Check sheet for the modelled part. Datum: model origin and axes. Units: mm. A direction names the side the tool comes from. Give positions to 0.01 mm unless a question says otherwise; leave off trailing zeros. Write each loop counter-clockwise with the first axis right and the second up, starting at its lowest first coordinate (ties: lowest second). Pieces come first, ordered by that corner, then holes. Notation, with made-up numbers: (26, 5) -> (81, 5) arc R17 cw to (81, 29) -> close; hole circle Ø6 at (88, 51). An arc over 180 degrees is marked (long way). Answer as a JSON object with one key per item and string values.
from build123d import *

# Parameters (mm, degrees)
F0_W     = 162.56
F0_H     = 120.65
F1_DEPTH = 6.35
F2_W     = 162.56
F2_H     = 120.65
F2_W_2   = 149.86
F2_H_2   = 107.95
F3_DEPTH = 6.35
F4_R     = 5.08


with BuildPart() as f1:
    # F0 (on Top) → F1 (new body)
    with BuildSketch(Plane.XY):
        with Locations((17.590381, -7.976995)):
            Rectangle(F0_W, F0_H)
    extrude(amount=F1_DEPTH)

    # F2 (on face) → F3 (join)
    with BuildSketch(Plane.XY.offset(6.35)):
        with Locations((17.590381, -7.976995)):
            Rectangle(F2_W, F2_H)
        with Locations((17.590381, -7.976995)):
            Rectangle(F2_W_2, F2_H_2, mode=Mode.SUBTRACT)
    extrude(amount=F3_DEPTH)

    # F4
    f4_edges = [f1.edges().sort_by_distance(p)[0] for p in [
        (98.870381, -68.301995, 6.35),
        (98.870381, 52.348005, 6.35),
        (-63.689619, 52.348005, 6.35),
        (-63.689619, -68.301995, 6.35),
    ]]
    fillet(f4_edges, radius=F4_R)


solid = f1.part
1. Scan lines: L1, parallel to X at y = -48.5, z = 7.5; L2, parallel to Y at x = 11.5, z = 12; L3, parallel to Z at x = 60, y = -47. Record each from-to range of solid material in increasing order. Write a range as [from, to].
Determined:
{"L1": "[-63.69, -57.34], [92.52, 98.87]", "L2": "[-68.3, -61.95], [46, 52.35]", "L3": "[0, 6.35]"}
2. Mould release check, pull along X, two halves, no side actions. Record for faces 1 (the face through (11, -66, 12.7)), 2 (the face through (-62.241, -66.774, 6.439)), 3 (the face through (92.52, -9, 9)): released by +X, released by -X, zero draft, split by the parting line, or undercut.
Determined:
{"face 1": "zero draft", "face 2": "released by -X", "face 3": "undercut"}
3. Go/stop test with a flat-tipped pin: P1, Ø2, axis at x = -25, y = 35, coming from the +Z side. Record where the tip stops, or that it passes through.
Determined:
{"P1": "z = 6.35"}
4. Access from +Z, -Z, +X, -X, +Y, -Y to the whole of each face (thin tool, end or side, straight path). Record for faces 4 (the face through (17, -61.952, 9)), 5 (the face through (17, 52.348, 6)).
Determined:
{"face 4": "+Z", "face 5": "+Z, -Z, +X, -X, +Y"}
5. Sectioned sample at C-C, the plane y = 24.5. Enter the section's corners in (x, z).
Determined:
{"outline": "(-63.69, 0) -> (98.87, 0) -> (98.87, 12.7) -> (92.52, 12.7) -> (92.52, 6.35) -> (-57.34, 6.35) -> (-57.34, 12.7) -> (-63.69, 12.7) -> close"}
6. Sectioned sample at A-A, the plane z = 8.25. Enter the section's corners in (x, y), plus the area to 3 significant figures.
Determined:
{"outline": "(-63.69, -63.22) arc R5.08 ccw to (-58.61, -68.3) -> (93.79, -68.3) arc R5.08 ccw to (98.87, -63.22) -> (98.87, 47.27) arc R5.08 ccw to (93.79, 52.35) -> (-58.61, 52.35) arc R5.08 ccw to (-63.69, 47.27) -> close; hole (-57.34, -61.95) -> (92.52, -61.95) -> (92.52, 46) -> (-57.34, 46) -> close", "area": "3,410 mm^2"}
7. Sectioned sample at B-B, the plane x = 71. Enter the section's corners in (y, z), plus the area to 3 significant figures.
Determined:
{"outline": "(-68.3, 0) -> (52.35, 0) -> (52.35, 12.7) -> (46, 12.7) -> (46, 6.35) -> (-61.95, 6.35) -> (-61.95, 12.7) -> (-68.3, 12.7) -> close", "area": "847 mm^2"}
